For this review, use the dimensioned drawing (mm, ordinates from the lowest corner) and the shaded views. A direction names the side the tool comes from. Give positions to 0.01 mm unless a question says otherwise; leave off trailing zeros. Order: outer loops, then holes, each group sorted by start corner. A loop starts at its lowest first (then second) coordinate and runs counter-clockwise, first axis right, second up.
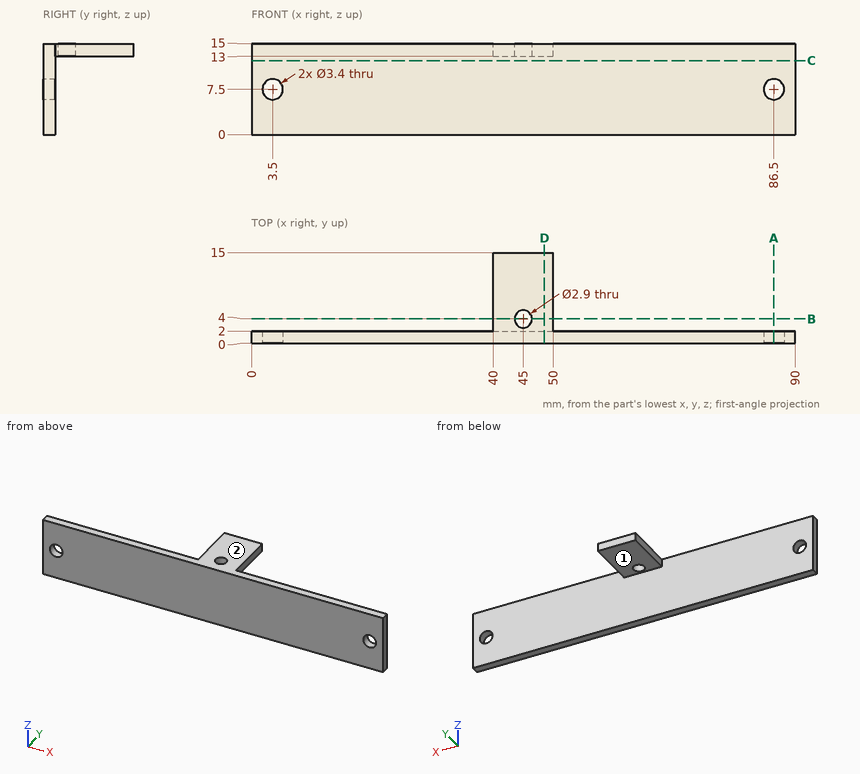
1. Take a section at D-D (x = 48.5). Write out the cut boundary in (y, z).
2. Insertion check: pin 1 (2 mm diameter, centred on x = 38.5, z = 9, fed in from -Y); pin 2 (2 mm diameter, centred on y = 10, z = 14, fed in from +X); pin 3 (3 mm diameter, centred on x = 13.5, z = 9, fed in from +Y); pin 4 (5 mm diameter, centred on x = 44.5, y = 5, fed in from -Z). Each pin has a flat end and moves straight along its axis. Give the tip position at first contact, or say it passes through.
3. Take a section at B-B (y = 4). Write out the cut boundary in (x, z).
4. Take a section at C-C (z = 12.25). Write out the cut boundary in (x, y), and give its area (3 significant figures).
5. To check wall thickness, follow line 1 (X direction, y = 1.2, z = 7.5); line 2 (Y direction, x = 45, z = 13.5); line 3 (Z direction, x = 86.5, y = 1.45). State the ranges of each line that lie inside material, in increasing order.
6. Take a section at A-A (x = 86.5). Write out the cut boundary in (y, z).
7. For the marked faces 1 and 2, list the 3-axis set-ups (+Z, -Z, +X, -X, +Y, -Y) from which the entire face can be reached by the end or side of a thin tool; tool diameter is ignored.
Answer:
1. outline: (0, 0) - (2, 0) - (2, 13) - (15, 13) - (15, 15) - (0, 15) - close
2. pin 1: stops at y = 0
2. pin 2: stops at x = 50
2. pin 3: stops at y = 2
2. pin 4: stops at z = 13
3. outline: (40, 13) - (43.55, 13) - (43.55, 15) - (40, 15) - close; (46.45, 13) - (50, 13) - (50, 15) - (46.45, 15) - close
4. outline: (0, 0) - (90, 0) - (90, 2) - (0, 2) - close
4. area: 180 mm2
5. line 1: x = 0 to 1.8, 5.2 to 84.8, 88.2 to 90
5. line 2: y = 0 to 2.55, 5.45 to 15
5. line 3: z = 0 to 5.8, 9.2 to 15
6. outline: (0, 0) - (2, 0) - (2, 5.8) - (0, 5.8) - close; (0, 9.2) - (2, 9.2) - (2, 15) - (0, 15) - close
7. face 1: -Z, +X, -X, +Y
7. face 2: +Z, +X, -X, +Y, -Y
